```python
from build123d import *

# Parameters (mm, degrees)
SKETCH_1_W          = 20
SKETCH_1_H          = 42.5
EXTRUDE_1_DEPTH     = 92.5
SKETCH_3_W          = 42.5
SKETCH_3_H          = 19
CUT_EXTRUDE_1_DEPTH = 5
FILLET_1_R          = 1


with BuildPart() as part:
    # 草图1 → 凸台-拉伸1 (new body)
    with BuildSketch(Plane(origin=(0, 0, 0), x_dir=(1, 0, 0), z_dir=(0, 1, 0))):
        Rectangle(SKETCH_1_W, SKETCH_1_H)
    extrude(amount=EXTRUDE_1_DEPTH)

    # 草图3 → 切除-拉伸1 (cut)
    with BuildSketch(Plane(origin=(10, 0, 0), x_dir=(0, 0, -1), z_dir=(1, 0, 0))):
        with Locations((0, 83)):
            Rectangle(SKETCH_3_W, SKETCH_3_H)
    extrude(amount=-CUT_EXTRUDE_1_DEPTH, mode=Mode.SUBTRACT)

    # 圆角1
    fillet_1_edges = [part.edges().sort_by_distance(p)[0] for p in [
        (-10, 92.5, 0),
        (-2.5, 92.5, -21.25),
        (10, 36.75, 21.25),
        (-2.5, 92.5, 21.25),
        (10, 36.75, -21.25),
        (5, 83, 21.25),
        (7.5, 73.5, 21.25),
        (5, 92.5, 0),
        (5, 83, -21.25),
        (5, 73.5, 0),
        (7.5, 73.5, -21.25),
        (10, 73.5, 0),
        (0, 0, 21.25),
        (-10, 0, 0),
        (0, 0, -21.25),
        (10, 0, 0),
        (-10, 46.25, 21.25),
        (-10, 46.25, -21.25),
    ]]
    fillet(fillet_1_edges, radius=FILLET_1_R)


solid = part.part
```
The model under review builds one solid part; all positions refer to its coordinate system, in mm. A direction names the side the tool comes from. Give positions to 0.01 mm unless a question says otherwise; leave off trailing zeros. Loops run counter-clockwise (first coordinate to the right, second up) from the corner with the lowest first, then second, coordinate; pieces in that order, holes last. Notation, with made-up numbers: (31, 61.5) -> (49, 61.5) arc R30 cw to (49, 99.5) -> close; hole circle Ø5 at (52.25, 20). An arc over 180 degrees is marked (long way). Use CSV: the item, a comma, the result in double quotes.
1. Consider section B-B, the plane y = 81. Write out the cut boundary in (x, z), then the cut area to 3 significant figures.
Result:
outline,"(-10, -20.25) arc R1 ccw to (-9, -21.25) -> (4, -21.25) arc R1 ccw to (5, -20.25) -> (5, 20.25) arc R1 ccw to (4, 21.25) -> (-9, 21.25) arc R1 ccw to (-10, 20.25) -> close"
area,"637 mm²"
2. For P1, Ø3.5, axis at x = 8, z = 4.5, coming from the +Y side; P2, Ø5, axis at y = 81.5, z = 6, coming from the +X side, all flat-tipped, find the tip position at first contact; note any pin that passes through.
Result:
P1,"stops at y = 73.5"
P2,"stops at x = 5"
3. Consider section C-C, the plane x = 8. Write out the cut boundary in (y, z), then the cut area to 3 significant figures.
Result:
outline,"(0, -20.25) arc R1 ccw to (1, -21.25) -> (72.5, -21.25) arc R1 ccw to (73.5, -20.25) -> (73.5, 20.25) arc R1 ccw to (72.5, 21.25) -> (1, 21.25) arc R1 ccw to (0, 20.25) -> close"
area,"3,120 mm²"
4. Consider section A-A, the plane z = -9. Write out the cut boundary in (x, y).
Result:
outline,"(-10, 1) arc R1 ccw to (-9, 0) -> (9, 0) arc R1 ccw to (10, 1) -> (10, 72.5) arc R1 ccw to (9, 73.5) -> (6, 73.5) arc R1 cw to (5, 74.5) -> (5, 91.5) arc R1 ccw to (4, 92.5) -> (-9, 92.5) arc R1 ccw to (-10, 91.5) -> close"
5. Machinability: for faces 1 (the face through (0, 46, -21.25)), 2 (the face through (8, 73.5, 0)), which of the approach directions +Z, -Z, +X, -X, +Y, -Y give a long, thin tool a straight path to every point of the face, cutting with its end or side? Answer none if there is none.
Result:
face 1,"-Z, +X, -X, +Y, -Y"
face 2,"+Z, -Z, +X, +Y"
6. To check wall thickness, follow probe 1 along X at (y, z) = (86.5, -1.5); probe 2 along Y at (x, z) = (5.75, 11.5); probe 3 along Z at (x, y) = (9.25, 49). State the ranges of each line that lie inside material, in increasing order. Write a range as from..to.
Result:
probe 1,"x = -10..5"
probe 2,"y = 0..73.53"
probe 3,"z = -21.22..21.22"
